from build123d import *

# Parameters (mm, degrees)
F0_W     = 50.8
F0_H     = 50.8
F1_DEPTH = 50.8
F2_W     = 25.4
F2_H     = 25.4
F3_DEPTH = 25.4
F4_W     = 25.4
F4_H     = 25.4
F5_DEPTH = 25.4
F6_R     = 15.835428
F7_DEPTH = 25.4
F8_R     = 14.993286
F9_DEPTH = 25.4


with BuildPart() as f1:
    # F0 (on Front) → F1 (new body)
    with BuildSketch(Plane.XZ):
        with Locations((-39.33969, 36.284415)):
            Rectangle(F0_W, F0_H)
    extrude(amount=F1_DEPTH)

    # F2 (on face) → F3 (join)
    with BuildSketch(Plane.XZ.offset(50.8)):
        with Locations((-39.33969, 36.951241)):
            Rectangle(F2_W, F2_H)
    extrude(amount=F3_DEPTH)

    # F4 (on face) → F5 (cut)
    with BuildSketch(Plane(origin=(-64.73969, 0, 0), x_dir=(0, -1, 0), z_dir=(-1, 0, 0))):
        with Locations((25.4, 37.333151)):
            Rectangle(F4_W, F4_H)
    extrude(amount=-F5_DEPTH, mode=Mode.SUBTRACT)

    # F6 (on face) → F7 (join)
    with BuildSketch(Plane.YZ.offset(-13.93969)):
        with Locations((-25.587924, 37.999976)):
            Circle(F6_R)
    extrude(amount=F7_DEPTH)

    # F8 (on face) → F9 (cut)
    with BuildSketch(Plane(origin=(0, 0, 0), x_dir=(-1, 0, 0), z_dir=(0, 1, 0))):
        with Locations((39.527614, 36.472339)):
            Circle(F8_R)
    extrude(amount=-F9_DEPTH, mode=Mode.SUBTRACT)


solid = f1.part
Input: part model. Units: mm. Frame: model coordinates. A direction names the side the tool comes from. Give positions to 0.01 mm unless a question says otherwise; leave off trailing zeros. Order: outer loops, then holes, each group sorted by start corner. A loop starts at its lowest first (then second) coordinate and runs counter-clockwise, first axis right, second up. Notation, with made-up numbers: (61.25, -16) - (79.25, -16) arc R22 ccw to (79.25, 20) - close; hole circle Ø4 at (35, 58). An arc over 180 degrees is marked (long way). Write each question's results on one line, items separated by ' | '.
Item 1: Section C-C (y = -30). Return loops of the section in (x, z), and give its area (3 significant figures).
A:
outline: (-64.74, 10.88) - (-13.94, 10.88) - (-13.94, 22.79) - (11.46, 22.79) - (11.46, 53.21) - (-13.94, 53.21) - (-13.94, 61.68) - (-64.74, 61.68) - (-64.74, 50.03) - (-39.34, 50.03) - (-39.34, 24.63) - (-64.74, 24.63) - close | area: 2,710 mm^2
Item 2: Contact query for flat-ended pins moving along their axis: pin 1 Ø12.5 at (y, z) = (-68.5, 41) entering from -X; pin 2 Ø6 at (x, z) = (-0.5, 40) entering from +Y; pin 3 Ø12 at (x, z) = (-38.5, 30) entering from +Y. Output: stop coordinate, or through.
A:
pin 1: stops at x = -52.04 | pin 2: stops at y = -9.75 | pin 3: stops at y = -25.4
Item 3: Section D-D (x = -41). Return loops of the section in (y, z), and give its area (3 significant figures).
A:
outline: (-76.2, 24.25) - (-50.8, 24.25) - (-50.8, 10.88) - (0, 10.88) - (0, 21.55) - (-25.4, 21.55) - (-25.4, 24.63) - (-38.1, 24.63) - (-38.1, 50.03) - (-25.4, 50.03) - (-25.4, 51.39) - (0, 51.39) - (0, 61.68) - (-50.8, 61.68) - (-50.8, 49.65) - (-76.2, 49.65) - close | area: 2,150 mm^2
Item 4: Section B-B (z = 32). Return loops of the section in (x, y), and give its area (3 significant figures).
A:
outline: (-64.74, -50.8) - (-52.04, -50.8) - (-52.04, -76.2) - (-26.64, -76.2) - (-26.64, -50.8) - (-13.94, -50.8) - (-13.94, -40.24) - (11.46, -40.24) - (11.46, -10.93) - (-13.94, -10.93) - (-13.94, 0) - (-25.22, 0) - (-25.22, -25.4) - (-39.34, -25.4) - (-39.34, -38.1) - (-64.74, -38.1) - close; (-64.74, -12.7) - (-53.84, -12.7) - (-53.84, 0) - (-64.74, 0) - close | area: 2,780 mm^2
Item 5: Access query for faces 4 (the flat face through (-52, -38.1, 37)), 5 (the flat face through (-39.34, -32, 38)), 6 (the flat face through (-52.04, -63, 37)). Directions: +Z, -Z, +X, -X, +Y, -Y. A direction counts if a zero-diameter tool reaches every point of the face in a straight line with its end or side. Return the directions, or none.
A:
face 4: -X | face 5: -X, +Y | face 6: +Z, -Z, -X, -Y
Item 6: Draft query along Y for faces 1 (the flat face through (-28, 0, 25)), 2 (the flat face through (-40, -25, 61.684)), 3 (the flat face through (-52, -25, 50.033)). Return one class per face: released by +Y, released by -Y, zero draft, split by the parting line, or undercut.
A:
face 1: released by +Y | face 2: zero draft | face 3: undercut
Item 7: Material intervals for line 1 along Z through (x, y) = (-59, -15); line 2 along Y through (x, z) = (-54, 31.5); line 3 along X through (y, z) = (-27.5, 18.5), sorted ascending.
A:
line 1: z = 10.88 to 24.63, 50.03 to 61.68 | line 2: y = -50.8 to -38.1, -12.7 to 0 | line 3: x = -64.74 to -13.94
Item 8: Section A-A (x = -58). Return loops of the section in (y, z).
A:
outline: (-50.8, 10.88) - (0, 10.88) - (0, 61.68) - (-50.8, 61.68) - close; hole (-38.1, 24.63) - (-12.7, 24.63) - (-12.7, 50.03) - (-38.1, 50.03) - close
